Autodesk Inventor part; units mm, degrees
ref_plane "YZ Plane" through (0, 0, 0) normal (1, 0, 0) x (0, 1, 0)
ref_plane "XZ Plane" through (0, 0, 0) normal (0, 1, 0) x (-1, 0, 0)
ref_plane "XY Plane" through (0, 0, 0) normal (0, 0, 1) x (1, 0, 0)
sketch "Sketch1" plane through (0, 0, 0) normal (0, 1, 0) x (-1, 0, 0)
  line L0 (-14.3889, -14.2778) -> (-11.3889, -14.2778)
  line L1 (-11.3889, -14.2778) -> (-11.3889, 54.2222)
  line L2 (-11.3889, 54.2222) -> (-14.3889, 54.2222)
  line L3 (-14.3889, 54.2222) -> (-14.3889, -14.2778)
  line L4 (-11.3889, 54.2222) -> (5.1111, 54.2222)
  line L5 (5.1111, 54.2222) -> (5.1111, 51.2222)
  line L6 (5.1111, 51.2222) -> (-11.3889, 51.2222)
  line L7 (-11.3889, 51.2222) -> (-11.3889, 54.2222)
  line L8 (5.1111, 54.2222) -> (8.1111, 54.2222)
  line L9 (8.1111, 54.2222) -> (8.1111, -14.2778)
  line L10 (8.1111, -14.2778) -> (5.1111, -14.2778)
  line L11 (5.1111, -14.2778) -> (5.1111, 54.2222)
  line L12 (8.1111, -14.2778) -> (18.1111, -14.2778)
  line L13 (18.1111, -14.2778) -> (18.1111, -11.2778)
  line L14 (18.1111, -11.2778) -> (8.1111, -11.2778)
  line L15 (8.1111, -11.2778) -> (8.1111, -14.2778)
  line L16 (-14.3889, -14.2778) -> (-24.3889, -14.2778)
  line L17 (-24.3889, -14.2778) -> (-24.3889, -11.2778)
  line L18 (-24.3889, -11.2778) -> (-14.3889, -11.2778)
  line L19 (-14.3889, -11.2778) -> (-14.3889, -14.2778)
  line L20 (-14.3889, 54.2222) -> (8.1111, 54.2222)
  line L21 (8.1111, 54.2222) -> (8.1111, 51.2222)
  line L22 (8.1111, 51.2222) -> (-14.3889, 51.2222)
  line L23 (-14.3889, 51.2222) -> (-14.3889, 54.2222)
  point P0 (0, 0)
  dimension "d0" = 10
  dimension "d1" = 10
  dimension "d2" = 3
  dimension "d3" = 3
  dimension "d4" = 3
  dimension "d5" = 3
  dimension "d6" = 3
  dimension "d7" = 68.5
  dimension "d8" = 16.5
extrude "Extrusion1" add sketch "Sketch1" along normal blind 10
sketch "Sketch2" plane through (14.3889, 0, 54.2222) normal (1, 0, 0) x (0, 0, -1)
  line L0 (0, 10) -> (65.5, 10)
  line L1 (0, 0) -> (65.5, 0)
  line L2 (31.75, 14.4261) -> (31.75, -5.3494)
  line L3 (68.5, 0) -> (68.5, 10)
  circle A0 centre (36.75, 4.5383) radius 2.25
  line L4 (31.75, 4.5383) -> (48.4854, 4.5383)
  point P0 (54.2222, 0)
  dimension "d11" = 36.75
  dimension "d12" = 4.5
  dimension "d13" = 5
extrude "Extrusion2" cut sketch "Sketch2" against normal blind 40
sketch "Sketch3" plane through (14.3889, 0, -11.2778) normal (0, 0, 1) x (1, 0, 0)
  circle A0 centre (5, 5) radius 2.25
  point P0 (-14.3889, 0)
  dimension "d16" = 4.5
extrude "Extrusion3" cut sketch "Sketch3" against normal blind 3
sketch "Sketch4" plane through (-18.1111, 0, -11.2778) normal (0, 0, 1) x (1, 0, 0)
  circle A0 centre (5, 5) radius 2.25
  point P0 (18.1111, 0)
  dimension "d19" = 4.5
extrude "Extrusion4" cut sketch "Sketch4" against normal blind 3
extrude "Extrusion5" add sketch "Sketch1" along normal blind 25 contours L22 L3 L2 L1 | L1 L4 L5 L6 | L5 L8 L9 L22
sketch "Sketch5" plane through (-8.1111, 0, 54.2222) normal (0, 0, 1) x (1, 0, 0)
  line L0 (0, 25) -> (22.5, 25)
  line L1 (0, 0) -> (0, 25)
  circle A0 centre (27.5, 5) radius 2.25
  line L2 (5.9472, 17) -> (15.4403, 17) construction
  line L3 (6.25, 22) -> (16.25, 22)
  line L4 (16.25, 22) -> (16.25, 12)
  line L5 (16.25, 12) -> (6.25, 12)
  line L6 (6.25, 12) -> (6.25, 22)
  line L7 (17.75, 23.5) -> (4.75, 23.5)
  line L8 (4.75, 23.5) -> (4.75, 10.5)
  line L9 (4.75, 10.5) -> (17.75, 10.5)
  line L10 (17.75, 10.5) -> (17.75, 23.5)
  point P0 (8.1111, 0)
  point P1 (11.25, 22)
  point P2 (11.25, 25)
  point P3 (16.25, 17)
  dimension "d24" = 12
  dimension "d25" = 10
  dimension "d26" = 10
  dimension "d27" = 1.5
extrude "Extrusion6" cut sketch "Sketch5" against normal blind 1 contours L10 L9 L8 L7
sketch "Sketch6" plane through (0, 0, 0) normal (0, 1, 0) x (-1, 0, 0)
  circle A0 centre (-13.3996, -12.6866) radius 5.8565
  circle A1 centre (6.9471, -12.6866) radius 6.4335
  point P0 (0, 0)
extrude "Extrusion7" add sketch "Sketch6" along normal blind 0.6
properties part number "BarClip"
Could you check a few things on this model? Use its own coordinates, in mm. A direction names the side the tool comes from. Round coordinates to 2 decimals unless told otherwise and drop trailing zeros. Order: outer loops, then holes, each group sorted by start corner. A loop starts at its lowest first (then second) coordinate and runs counter-clockwise, first axis right, second up. Notation, with made-up numbers: (33, -20) -> (52, -20) arc R26 cw to (52, -3) -> close; hole circle Ø8 at (63.25, 47). An arc over 180 degrees is marked (long way). One line per question, with ' | ' between items.
Q1. I'm going to push flat-ended pins straight in: pin 1 (5 mm diameter, centred on y = 10.5, z = 12, fed in from +X); pin 2 (11 mm diameter, centred on y = 7, z = 19.5, fed in from -X); pin 3 (6 mm diameter, centred on x = 0, y = 4, fed in from -Z). Where does each tip first touch, or does it pass through?
Computed values:
pin 1: x = 14.39 | pin 2: x = -8.11 | pin 3: z = 51.22
Q2. Which directions (+Z, -Z, +X, -X, +Y, -Y) give clear straight access to the entire face, cutting with the end or side of a thin tool? Please do faces 4 (the face through (3, 17, 54.222)), 5 (the face through (-7, 10, 16)), 6 (the face through (-2.626, 0.296, -17.453)), 7 (the face through (-10, 0.6, -9)), 8 (the face through (16, 0.6, -10)).
Computed values:
face 4: +Z, +X, -X, +Y, -Y | face 5: -Z, +X, -X, +Y | face 6: +Y, -Y | face 7: +Z, -X, +Y | face 8: +Z, +X, +Y
Q3. If we section it at A-A on z = 30: Write out the boundary of the cut face in (x, y).
Computed values:
outline: (-8.11, 0) -> (-5.11, 0) -> (-5.11, 10) -> (-8.11, 10) -> close; (11.39, 0) -> (14.39, 0) -> (14.39, 10) -> (11.39, 10) -> close
Q4. If we section it at B-B on x = -7: Write out the boundary of the cut face in (y, z), plus the area to 3 significant figures.
Computed values:
outline: (0, -19.12) -> (0.6, -19.12) -> (0.6, -14.28) -> (10, -14.28) -> (10, 51.22) -> (25, 51.22) -> (25, 54.22) -> (0, 54.22) -> close; hole circle Ø4.5 at (4.54, 17.47) | area: 717 mm²
Q5. If we section it at C-C on x = 15.5: Write out the boundary of the cut face in (y, z).
Computed values:
outline: (0, -18.15) -> (0.6, -18.15) -> (0.6, -14.28) -> (10, -14.28) -> (10, -11.28) -> (0.6, -11.28) -> (0.6, -7.22) -> (0, -7.22) -> close
Q6. We'd pull the mould along Z, two halves only. Please class faces 1 (the face through (12.91, 4.64, 19.72)), 2 (the face through (3, 10, 54.222)), 3 (the face through (16.5, 4.9, -14.278)): released by +Z, released by -Z, zero draft, split by the parting line, or undercut.
Computed values:
face 1: undercut | face 2: released by +Z | face 3: released by -Z
Q7. If I drill on line 1 (X direction, y = 9, z = 34); line 2 (Z direction, x = 11, y = 12.75); line 3 (Y direction, x = 14, z = 11.5), over which ranges is the centre line in solid material (lowest first)? Write a range as from..to.
Computed values:
line 1: -8.11..-5.11, 11.39..14.39 | line 2: 51.22..54.22 | line 3: 0..10
